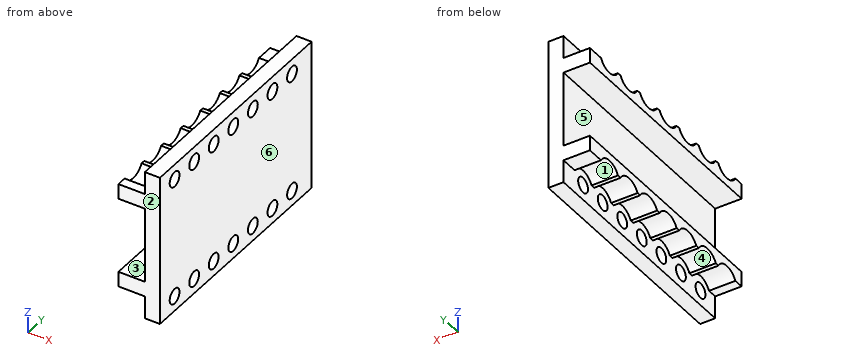
from build123d import *

# Parameters (mm, degrees)
PAD028_DEPTH    = 62
SKETCH049_W     = 40
SKETCH049_H     = 62
PAD029_DEPTH    = 4
SKETCH009_R     = 2
POCKET017_DEPTH = 4
SKETCH010_R     = 4
POCKET018_DEPTH = 7


with BuildPart() as leftmiddle:
    # Sketch048 → Pad028 (new body)
    with BuildSketch(Plane.XZ):
        Polygon((0, 0), (0, 10), (7, 10), (7, 14), (-4, 14), (-4, -14), (7, -14), (7, -10), (0, -10), align=None)
    extrude(amount=PAD028_DEPTH)

    # Sketch049 (on Face4 of Pad028) → Pad029 (join)
    with BuildSketch(Plane(origin=(-4, 0, 0), x_dir=(0, 0, -1), z_dir=(-1, 0, 0))):
        with Locations((0, 31)):
            Rectangle(SKETCH049_W, SKETCH049_H)
    extrude(amount=-PAD029_DEPTH)

    # Sketch009 (on Face14 of Pad029) → Pocket017 (cut)
    with BuildSketch(Plane(origin=(-4, 0, 0), x_dir=(0, 0, -1), z_dir=(-1, 0, 0))):
        with Locations((-16, 8)):
            Circle(SKETCH009_R)
        with Locations((-16, 16)):
            Circle(SKETCH009_R)
        with Locations((-16, 24)):
            Circle(SKETCH009_R)
        with Locations((-16, 32)):
            Circle(SKETCH009_R)
        with Locations((-16, 40)):
            Circle(SKETCH009_R)
        with Locations((-16, 48)):
            Circle(SKETCH009_R)
        with Locations((-16, 56)):
            Circle(SKETCH009_R)
        with Locations((16, 56)):
            Circle(SKETCH009_R)
        with Locations((16, 48)):
            Circle(SKETCH009_R)
        with Locations((16, 40)):
            Circle(SKETCH009_R)
        with Locations((16, 32)):
            Circle(SKETCH009_R)
        with Locations((16, 24)):
            Circle(SKETCH009_R)
        with Locations((16, 16)):
            Circle(SKETCH009_R)
        with Locations((16, 8)):
            Circle(SKETCH009_R)
    extrude(amount=-POCKET017_DEPTH, mode=Mode.SUBTRACT)

    # Sketch010 (on Face14 of Pocket017) → Pocket018 (cut)
    with BuildSketch(Plane(origin=(0, 0, 0), x_dir=(0, 0, 1), z_dir=(1, 0, 0))):
        with Locations((-16, 8)):
            Circle(SKETCH010_R)
        with Locations((-16, 16)):
            Circle(SKETCH010_R)
        with Locations((-16, 24)):
            Circle(SKETCH010_R)
        with Locations((-16, 32)):
            Circle(SKETCH010_R)
        with Locations((-16, 40)):
            Circle(SKETCH010_R)
        with Locations((-16, 48)):
            Circle(SKETCH010_R)
        with Locations((-16, 56)):
            Circle(SKETCH010_R)
        with Locations((16, 56)):
            Circle(SKETCH010_R)
        with Locations((16, 48)):
            Circle(SKETCH010_R)
        with Locations((16, 40)):
            Circle(SKETCH010_R)
        with Locations((16, 32)):
            Circle(SKETCH010_R)
        with Locations((16, 24)):
            Circle(SKETCH010_R)
        with Locations((16, 16)):
            Circle(SKETCH010_R)
        with Locations((16, 8)):
            Circle(SKETCH010_R)
    extrude(amount=POCKET018_DEPTH, mode=Mode.SUBTRACT)


with BuildPart() as leftmiddle_1:
    # Body015 placement: moved
    add(leftmiddle.part.moved(Location((-92, -203.5, 13.5))))


with BuildPart() as rightmiddle:
    # Part__Mirroring005: instance of LeftMiddle
    add(leftmiddle_1.part.mirror(Plane(origin=(0, 0, 0), x_dir=(0, -1, 0), z_dir=(1, 0, 0))))


solid = rightmiddle.part
Could you check a few things on this model? Use its own coordinates, in mm. Face numbers are marked on the shaded views. A direction names the side the tool comes from. Give positions to 0.01 mm unless a question says otherwise; leave off trailing zeros. Loops run counter-clockwise (first coordinate to the right, second up) from the corner with the lowest first, then second, coordinate; pieces in that order, holes last. Notation, with made-up numbers: M -23,-18.75 L 24,-18.75 A24 cw 24,7.25 Z; hole C 6.5,-10.75 d5. An arc over 180 degrees is marked long. Answer as a JSON object with one key per item and string values.
Q1. For the marked faces 4, 5 and 6, which set-ups out of +Z, -Z, +X, -X, +Y, -Y let a thin tool reach every point of the face, with its end or its side?
Values found:
{"face 4": "-Z, -X", "face 5": "-X, +Y, -Y", "face 6": "+Z, -Z, +X, +Y, -Y"}
Q2. If we mould it in two halves opening along Y, with no side actions, what happens to the marked faces 1, 2 and 3? For each: pulls with the +Y half, pulls with the -Y half, needs draft (parallel to the pull), parting line crosses it, or undercut.
Values found:
{"face 1": "undercut", "face 2": "pulls with the -Y half", "face 3": "needs draft"}
Q3. If I drill on probe 1 along Z at (x, y) = (93.7, -243.5); probe 2 along Z at (x, y) = (89.75, -259.5); probe 3 along X at (y, z) = (-217.5, 5.5), over which ranges is the centre line in solid material (lowest first)? Write a range as [from, to].
Values found:
{"probe 1": "z = [-6.5, -4.5], [-0.5, 27.5], [31.5, 33.5]", "probe 2": "z = [1.5, 3.5], [23.5, 25.5]", "probe 3": "x = [92, 96]"}
Q4. For P1, Ø5, axis at y = -219.5, z = -2.5, coming from the -X side; P2, Ø2.5, axis at x = 89.5, y = -205, coming from the +Z side; P3, Ø3, axis at x = 89.5, y = -264, coming from the -Z side, each with a flat end and sliding along its axis, tell me the tip position at first contact or that it passes through.
Values found:
{"P1": "stops at x = 92", "P2": "stops at z = 27.5", "P3": "stops at z = -0.5"}
Q5. Suppose I cut it at C-C, the plane y = -219.5. List the corners of the cut face in (x, z) for me.
Values found:
{"outline": "M 85,1.5 L 92,1.5 L 92,-0.5 L 96,-0.5 L 96,27.5 L 92,27.5 L 92,25.5 L 85,25.5 L 85,23.5 L 92,23.5 L 92,3.5 L 85,3.5 Z; M 92,-6.5 L 96,-6.5 L 96,-4.5 L 92,-4.5 Z; M 92,31.5 L 96,31.5 L 96,33.5 L 92,33.5 Z"}
Q6. Suppose I cut it at A-A, the plane x = 93.75. State how many separate pieces and enclosed holes the cut face has, plus the area to 3 significant figures.
Values found:
{"separate pieces": "1", "enclosed holes": "14", "area": "2,300 mm²"}
Q7. Suppose I cut it at D-D, the plane z = 5. List the corners of the cut face in (x, y) for me.
Values found:
{"outline": "M 92,-265.5 L 96,-265.5 L 96,-203.5 L 92,-203.5 Z"}
